from build123d import *

# Parameters (mm, degrees)
BOSS_EXTRUDE1_DEPTH   = 12.6
SKETCH2_R             = 5.0000000000000036
CUT_EXTRUDE1_DEPTH    = 48.150424176246815
SKETCH3_W             = 10.00000000000001
SKETCH3_H             = 10.000000000000007
CUT_EXTRUDE2_DEPTH    = 11.6
CHAMFER1_SIZE         = 5
CHAMFER1_SIZE2        = 11.230183869521158
CUT_EXTRUDE3_DEPTH    = 48.150424176246815
BOSS_EXTRUDE2_DEPTH   = 40
SKETCH6_R             = 1.7500000000000004
SKETCH6_R_2           = 1.7500000000000002
BOSS_EXTRUDE3_DEPTH   = 3
CUT_EXTRUDE4_DEPTH    = 48.369406002186686
CUT_EXTRUDE5_DEPTH    = 47.07236166447865
BOSS_EXTRUDE4_DEPTH   = 6
SKETCH12_R            = 1.4000000000000001
CUT_EXTRUDE6_DEPTH    = 38.90502227131958
BOSS_EXTRUDE5_REACH   = 44.93
SKETCH14_W            = 3.5000000000000036
SKETCH14_H            = 3.265431857231029
CUT_EXTRUDE7_REACH    = 46.879
CUT_EXTRUDE8_REACH    = 46.879
M2_TAPPED_HOLE1_D     = 1.6
M2_TAPPED_HOLE1_DEPTH = 4.2
M2_TAPPED_HOLE1_TIP   = 0.48068849522204826
FILLET1_R             = 1
FILLET2_R             = 2
FILLET4_R             = 2


with BuildPart() as part:
    # Sketch1 → Boss-Extrude1 (new body)
    with BuildSketch(Plane.XY):
        Polygon((0, 0), (40, 0), (39.99999999999999, 21.550000000000004), (0, 21.550000000000004), align=None)
    extrude(amount=BOSS_EXTRUDE1_DEPTH)

    # Sketch2 → Cut-Extrude1 (cut, through all)
    with BuildSketch(Plane.XY.offset(12.6)):
        with Locations((19.999999999999996, 10.775000000000004)):
            Circle(SKETCH2_R)
    extrude(amount=-CUT_EXTRUDE1_DEPTH, mode=Mode.SUBTRACT)

    # Sketch3 → Cut-Extrude2 (cut)
    with BuildSketch(Plane.XY.offset(12.6)):
        with Locations((20, 10.775000000000002)):
            Rectangle(SKETCH3_W, SKETCH3_H)
    extrude(amount=-CUT_EXTRUDE2_DEPTH, mode=Mode.SUBTRACT)

    # Chamfer1
    chamfer1_edges = [part.edges().sort_by_distance(p)[0] for p in [
        (14.999999999999993, 10.775000000000002, 12.6),
        (19.999999999999996, 5.7749999999999995, 12.6),
        (25, 10.775000000000004, 12.6),
    ]]
    chamfer1_side = [part.faces().sort_by_distance(p)[0] for p in [
        (20, 0.45435696319083746, 12.6),
    ]]
    chamfer(chamfer1_edges, length=CHAMFER1_SIZE, length2=CHAMFER1_SIZE2, reference=chamfer1_side[0])

    # Sketch4 → Cut-Extrude3 (cut, through all)
    with BuildSketch(Plane.ZY):
        Polygon((12.6, 0), (5.164224911806891, 20.42962415095372), (0, 18.550000000000004), (0, 21.550000000000004), (12.6, 21.550000000000004), align=None)
    extrude(amount=-CUT_EXTRUDE3_DEPTH, mode=Mode.SUBTRACT)

    # Sketch5 → Boss-Extrude2 (add)
    with BuildSketch(Plane.ZY):
        Polygon((12.6, 0), (0, -4.5860249517541645), (0, 0), align=None)
    extrude(amount=-BOSS_EXTRUDE2_DEPTH)

    # Sketch6 → Boss-Extrude3 (add)
    with BuildSketch(Plane.XY.offset(-2.9999999999999996)):
        with Locations(Location((19.999999999999996, 20.275000000000002, 0), (0, 0, 260.303678946))):
            Circle(SKETCH6_R)
        with Locations(Location((20, 1.275000000000002, 0), (0, 0, 180))):
            Circle(SKETCH6_R_2)
    extrude(amount=BOSS_EXTRUDE3_DEPTH)

    # Sketch7 → Cut-Extrude4 (cut, through all)
    with BuildSketch(Plane(origin=(40, 1.288e-14, 0), x_dir=(0, 0, -1), z_dir=(1, 3.2e-16, 0))):
        Polygon((0, -4.586024951754178), (0, -0.47500000000000464), (-1.3212579510498954, -4.105126385784462), align=None)
    extrude(amount=-CUT_EXTRUDE4_DEPTH, mode=Mode.SUBTRACT)

    # Sketch8 → Cut-Extrude5 (cut, through all)
    with BuildSketch(Plane(origin=(0, 4.049561941025207, 11.126079991649561), x_dir=(1, 0, 0), z_dir=(0, 0.34202014332566943, 0.9396926207859082))):
        Polygon((0, 17.4312981155786), (9.149876173671583, 17.4312981155786), (9.149876173671586, -4.309453805903435), (0, -4.309453805903436), align=None)
        Polygon((40, -4.309453805903436), (30.850123826328417, -4.309453805903435), (30.850123826328417, 17.4312981155786), (40, 17.4312981155786), align=None)
    extrude(amount=-CUT_EXTRUDE5_DEPTH, mode=Mode.SUBTRACT)

    # Sketch11 → Boss-Extrude4 (add)
    with BuildSketch(Plane.ZY.offset(-9.149876173671585)):
        Polygon((4.8e-16, 18.550000000000008), (1.879385241571817, 19.234040286651346), (3.9315061015258332, 13.595884561935897), (2.0521208599540164, 12.911844275284558), align=None)
    boss_extrude4 = extrude(amount=BOSS_EXTRUDE4_DEPTH)

    # Sketch12 → Cut-Extrude6 (cut, through all)
    with BuildSketch(Plane(origin=(0, 2.8539780767228278, 7.841240321414484), x_dir=(1, 0, 0), z_dir=(0, 0.3420201433256694, 0.9396926207859083))):
        with Locations(Location((6.149876173671584, 14.431298115578603, 0), (0, 0, 270))):
            Circle(SKETCH12_R)
    cut_extrude6 = extrude(amount=-CUT_EXTRUDE6_DEPTH, mode=Mode.SUBTRACT)

    # Mirror1: Boss-Extrude4, Cut-Extrude6 across plane
    add(boss_extrude4.mirror(Plane.ZY.offset(-19.999999999999996)))
    add(cut_extrude6.mirror(Plane.ZY.offset(-19.999999999999996)), mode=Mode.SUBTRACT)

    # Boss-Extrude5: up to this plane
    boss_extrude5_end = Plane(origin=(0, 0, 0), z_dir=(0, 0, -1))
    # Sketch14 → Boss-Extrude5 (add, up to the surface)
    with BuildSketch(Plane(origin=(0, 2.8539780767228278, 7.841240321414484), x_dir=(1, 0, 0), z_dir=(0, 0.3420201433256694, 0.9396926207859083)), mode=Mode.PRIVATE) as boss_extrude5_sk1:
        with Locations((20, 19.064014044194117)):
            Rectangle(SKETCH14_W, SKETCH14_H)
    boss_extrude5_tool1 = split(extrude(boss_extrude5_sk1.sketch, amount=-BOSS_EXTRUDE5_REACH, mode=Mode.PRIVATE), bisect_by=boss_extrude5_end, keep=Keep.BOTH, mode=Mode.PRIVATE)
    add(boss_extrude5_tool1.solids().sort_by_distance((20, 20.768291, 1.320964))[0])

    # Cut-Extrude7: up to this plane
    cut_extrude7_end = Plane(origin=(0, 2.8539780767228256, 7.841240321414483), z_dir=(0, -0.3420201433256692, -0.9396926207859083))
    # Sketch15 → Cut-Extrude7 (cut, up to the surface)
    with BuildSketch(Plane(origin=(0, 0, 0), x_dir=(-1, 0, 0), z_dir=(0, 0, -1)), mode=Mode.PRIVATE) as cut_extrude7_sk1:
        with BuildLine():
            Line((-19.999999999999996, 22.025000000000006), (-21.75, 22.02500000000001))
            Line((-21.75, 22.02500000000001), (-21.750000000000004, 20.275000000000002))
            ThreePointArc((-21.750000000000004, 20.275000000000002), (-21.237436867076458, 21.512436867076463), (-19.999999999999996, 22.025000000000006))
        make_face()
    cut_extrude7_tool1 = split(extrude(cut_extrude7_sk1.sketch, amount=-CUT_EXTRUDE7_REACH, mode=Mode.PRIVATE), bisect_by=cut_extrude7_end, keep=Keep.BOTH, mode=Mode.PRIVATE)
    add(cut_extrude7_tool1.solids().sort_by_distance((21.359106, 21.634106, 0))[0], mode=Mode.SUBTRACT)

    # Cut-Extrude8: up to this plane
    cut_extrude8_end = Plane(origin=(0, 2.8539780767228256, 7.841240321414483), z_dir=(0, -0.3420201433256692, -0.9396926207859083))
    # Sketch16 → Cut-Extrude8 (cut, up to the surface)
    with BuildSketch(Plane(origin=(0, 0, 0), x_dir=(-1, 0, 0), z_dir=(0, 0, -1)), mode=Mode.PRIVATE) as cut_extrude8_sk1:
        with BuildLine():
            Line((-18.249999999999993, 20.275000000000002), (-18.249999999999996, 22.02500000000001))
            Line((-18.249999999999996, 22.02500000000001), (-19.999999999999996, 22.025000000000006))
            ThreePointArc((-19.999999999999996, 22.025000000000006), (-18.762563132923535, 21.512436867076463), (-18.249999999999993, 20.275000000000002))
        make_face()
    cut_extrude8_tool1 = split(extrude(cut_extrude8_sk1.sketch, amount=-CUT_EXTRUDE8_REACH, mode=Mode.PRIVATE), bisect_by=cut_extrude8_end, keep=Keep.BOTH, mode=Mode.PRIVATE)
    add(cut_extrude8_tool1.solids().sort_by_distance((18.640894, 21.634106, 0))[0], mode=Mode.SUBTRACT)


with BuildPart() as body_2:
    # of the pieces the cut leaves, the one that is kept (cut_extrude8_keep)
    add(part.part.solids().sort_by_distance((30.850123826, -0.475, 0))[0])

    # M2 Tapped Hole1
    with Locations(Plane(origin=(20, 20.275, -3), x_dir=(-1, 0, 0), z_dir=(0, 0, -1))):
        with Locations((0, 0), (0, -19)):
            Hole(M2_TAPPED_HOLE1_D / 2, depth=M2_TAPPED_HOLE1_DEPTH)
            with Locations((0, 0, -(M2_TAPPED_HOLE1_DEPTH + M2_TAPPED_HOLE1_TIP / 2))):  # 118° drill point
                Cone(0, M2_TAPPED_HOLE1_D / 2, M2_TAPPED_HOLE1_TIP, mode=Mode.SUBTRACT)

    # Fillet1
    fillet1_edges = [body_2.edges().sort_by_distance(p)[0] for p in [
        (18.249999999999996, 18.89202014332568, 0.9396926207859103),
        (21.75, 18.89202014332568, 0.9396926207859103),
        (36.85012382632841, 18.892020143325677, 0.9396926207859077),
        (30.850123826328407, 13.253864418610231, 2.9918134807399235),
        (9.149876173671583, 13.25386441861023, 2.9918134807399244),
        (3.149876173671583, 13.253864418610227, 2.991813480739925),
        (3.149876173671582, 18.892020143325677, 0.9396926207859085),
        (36.85012382632841, 13.253864418610231, 2.991813480739924),
    ]]
    fillet(fillet1_edges, radius=FILLET1_R)

    # Fillet2
    fillet2_edges = [body_2.edges().sort_by_distance(p)[0] for p in [
        (9.149876173671586, -2.052563192892223, 6.960628975524948),
        (9.149876173671583, 19.831832218802536, 3.521805076689357),
        (30.850123826328417, -2.0525631928922223, 6.9606289755249495),
        (30.850123826328417, 19.831832218802536, 3.5218050766893576),
    ]]
    fillet(fillet2_edges, radius=FILLET2_R)

    # Fillet4
    fillet4_edges = [body_2.edges().sort_by_distance(p)[0] for p in [
        (26.22183071260031, 15.775000000000007, 4.114092842464741),
    ]]
    fillet(fillet4_edges, radius=FILLET4_R)
    fillet4_2_edges = [body_2.edges().sort_by_distance(p)[0] for p in [
        (13.778169287399688, 15.775000000000006, 4.114092842464743),
    ]]
    fillet(fillet4_2_edges, radius=FILLET4_R)
    fillet4_3_edges = [body_2.edges().sort_by_distance(p)[0] for p in [
        (14.999999999999993, 15.775000000000007, 1.184908065239421),
    ]]
    fillet(fillet4_3_edges, radius=FILLET4_R)
    fillet4_4_edges = [body_2.edges().sort_by_distance(p)[0] for p in [
        (25, 15.775000000000007, 1.184908065239421),
    ]]
    fillet(fillet4_4_edges, radius=FILLET4_R)
    fillet4_5_edges = [body_2.edges().sort_by_distance(p)[0] for p in [
        (12.574938086835799, 3.3499380868358024, 6.81659436644018),
    ]]
    fillet(fillet4_5_edges, radius=FILLET4_R)
    fillet4_6_edges = [body_2.edges().sort_by_distance(p)[0] for p in [
        (27.425061913164196, 3.349938086835803, 6.816594366440178),
    ]]
    fillet(fillet4_6_edges, radius=FILLET4_R)
    fillet4_7_edges = [body_2.edges().sort_by_distance(p)[0] for p in [
        (25, 5.7749999999999995, 1.7667114299152384),
    ]]
    fillet(fillet4_7_edges, radius=FILLET4_R)
    fillet4_8_edges = [body_2.edges().sort_by_distance(p)[0] for p in [
        (14.999999999999993, 5.7749999999999995, 1.766711429915226),
    ]]
    fillet(fillet4_8_edges, radius=FILLET4_R)


solid = body_2.part
Source: CAD feature listing. Evaluate the final solid. Frame: model axes, mm. A direction names the side the tool comes from. Give positions to 0.01 mm unless a question says otherwise; leave off trailing zeros. Order: outer loops, then holes, each group sorted by start corner. A loop starts at its lowest first (then second) coordinate and runs counter-clockwise, first axis right, second up. Notation, with made-up numbers: (26.5, 65.25) -> (82.5, 65.25) arc R29 ccw to (82.5, 85.25) -> close; hole circle Ø1 at (36, 11.5). An arc over 180 degrees is marked (long way). Use a Markdown table: item, result.
1) Ray query, line 1 along Y through (x, z) = (20, -1.2) (3 decimals); line 2 along X through (y, z) = (3.25, 3.5); line 3 along X through (y, z) = (4.5, 9.5). Return the intervals inside material, ascending. Write a range as [from, to].
Answer list:
| item | result |
|---|---|
| line 1 | [-0.475, 0.475], [2.075, 3.025], [18.525, 19.475], [21.075, 22.025] |
| line 2 | [9.15, 30.85] |
| line 3 | [9.15, 11.38], [28.62, 30.85] |
2) Contact query for flat-ended pins moving along their axis: P1, Ø5.5, axis at x = 22, y = 14.5, coming from the +Z side; P2, Ø5.5, axis at x = 16.5, y = 7.5, coming from the +Z side; P3, Ø1, axis at x = 10, z = 1.5, coming from the -Y side. Output: stop coordinate, or through.
Answer list:
| item | result |
|---|---|
| P1 | z = 6.86 |
| P2 | z = 4.18 |
| P3 | y = -3.99 |
3) Mould query, pull axis X, two halves, no side actions, for faces 1 (the flat face through (12.787, 9.551, 6.341)), 2 (the flat face through (19.876, -2.024, 7.04)), 3 (the cylindrical face through (19.18, 21.82, -1.28)). Classes: +X half, -X half, draft (parallel to the pull), parting line (faces both ways), or undercut.
Answer list:
| item | result |
|---|---|
| face 1 | undercut |
| face 2 | draft |
| face 3 | parting line |
4) Reachability of faces 4 (the flat face through (16.2, 14.4, 1)), 5 (the cylindrical face through (9.751, -1.545, 6.687)), 6 (the cylindrical face through (21.75, 1.2, -1.52)), 7 (the cylindrical face through (30.28, 19.258, 3.705)), 8 (the flat face through (19.35, 20.339, 1.477)) from +Z, -Z, +X, -X, +Y, -Y: full face, straight path, thin tool, end or side. Return the list, or none.
Answer list:
| item | result |
|---|---|
| face 4 | +Z |
| face 5 | +Z, -X, -Y |
| face 6 | -Z |
| face 7 | +X, +Y |
| face 8 | +X, -X, +Y |
5) Section query A-A, the plane y = 9.75. Return the cut outline in (x, z), then the cut area to 3 significant figures.
Answer list:
| item | result |
|---|---|
| outline | (9.15, 0) -> (15.11, 0) -> (15.11, 1) -> (15, 1) -> (15, 1.37) -> (11.58, 9.05) -> (9.15, 9.05) -> close; (24.89, 0) -> (30.85, 0) -> (30.85, 9.05) -> (28.42, 9.05) -> (25, 1.37) -> (25, 1) -> (24.89, 1) -> close |
| area | 79.8 mm² |
